Input: part model. Units: mm. Frame: model coordinates. Face numbers are marked on the shaded views. Round coordinates to 2 decimals unless told otherwise and drop trailing zeros. Write each loop counter-clockwise with the first axis right and the second up, starting at its lowest first coordinate (ties: lowest second). Pieces come first, ordered by that corner, then holes. Notation, with made-up numbers: (57.25, 86.25) -> (72.25, 86.25) arc R21 ccw to (72.25, 119.25) -> close; hole circle Ø9 at (-5.5, 19). An arc over 180 degrees is marked (long way). Write item = value, one per line.
```python
from build123d import *

# Parameters (mm, degrees)
SKETCH1_R           = 25
BOSS_EXTRUDE1_DEPTH = 29.5
SKETCH2_R           = 40
BOSS_EXTRUDE2_DEPTH = 3
CHAMFER1_SIZE       = 1
SKETCH3_R           = 21
CUT_EXTRUDE1_DEPTH  = 26
FILLET1_R           = 0.5
SKETCH4_R           = 2
CUT_EXTRUDE2_DEPTH  = 26
CIRPATTERN1_COUNT   = 4
CHAMFER2_SIZE       = 0.5


with BuildPart() as part:
    # Sketch1 → Boss-Extrude1 (new body)
    with BuildSketch(Plane.XY):
        Circle(SKETCH1_R)
    extrude(amount=BOSS_EXTRUDE1_DEPTH)

    # Sketch2 → Boss-Extrude2 (add)
    with BuildSketch(Plane.XY.offset(29.5)):
        Circle(SKETCH2_R)
    extrude(amount=-BOSS_EXTRUDE2_DEPTH)

    # Chamfer1
    chamfer1_edges = [part.edges().sort_by_distance(p)[0] for p in [
        (-25, 0, 0),
        (-25, 0, 26.5),
    ]]
    chamfer(chamfer1_edges, length=CHAMFER1_SIZE)

    # Sketch3 → Cut-Extrude1 (cut)
    with BuildSketch(Plane.XY.offset(29.5)):
        Circle(SKETCH3_R)
    extrude(amount=-CUT_EXTRUDE1_DEPTH, mode=Mode.SUBTRACT)

    # Fillet1
    fillet1_edges = [part.edges().sort_by_distance(p)[0] for p in [
        (-40, 0, 26.5),
        (-40, 0, 29.5),
    ]]
    fillet(fillet1_edges, radius=FILLET1_R)

    # Sketch4 → Cut-Extrude2 (cut)
    with BuildSketch(Plane(origin=(0, 0, 26.5), x_dir=(-1, 0, 0), z_dir=(0, 0, -1))):
        with Locations((0, 32.5)):
            Circle(SKETCH4_R)
    cut_extrude2 = extrude(amount=-CUT_EXTRUDE2_DEPTH, mode=Mode.SUBTRACT)

    # CirPattern1: Cut-Extrude2 ×4 about axis
    cirpattern1_axis = Axis((0, 0, 0), (0, 0, 1))
    for i in range(1, CIRPATTERN1_COUNT):
        add(cut_extrude2.rotate(cirpattern1_axis, i * 360 / CIRPATTERN1_COUNT), mode=Mode.SUBTRACT)

    # Chamfer2
    chamfer2_edges = [part.edges().sort_by_distance(p)[0] for p in [
        (2, 32.5, 26.5),
        (32.5, -2, 26.5),
        (-2, -32.5, 29.5),
        (-2, -32.5, 26.5),
        (-32.5, 2, 26.5),
    ]]
    chamfer(chamfer2_edges, length=CHAMFER2_SIZE)


solid = part.part
```
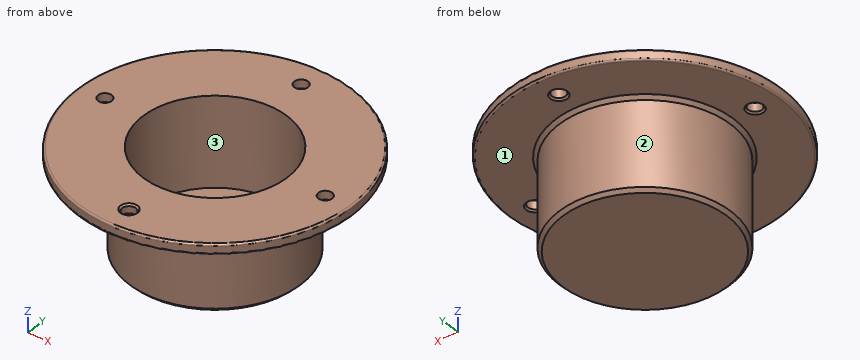
1) Line query: L1, parallel to Y at x = 0, z = 28; L2, parallel to Y at x = -0.5, z = 27.25; L3, parallel to Z at x = -15, y = -4. Output: solid intervals per line, ascending. Write a range as from..to.
Solutions:
L1 = -40..-34.5, -30.5..-21, 21..30.5, 34.5..40
L2 = -40..-34.44, -30.56..-20.99, 20.99..30.56, 34.44..40
L3 = 0..3.5
2) Draft query along Y for the marked faces 1, 2 and 3. Return one class per face: +Y half, -Y half, draft (parallel to the pull), parting line (faces both ways), or undercut.
Solutions:
face_1 = draft
face_2 = parting line
face_3 = undercut
3) First-contact query: P1, Ø5, axis at x = 2, z = 9, coming from the -Y side; P2, Ø6.5, axis at x = 0, y = -32.5, coming from the -Z side; P3, Ø3, axis at x = 32.5, y = 0, coming from the -Z side; P4, Ø8, axis at y = 26.5, z = 4, coming from the +X side. Flat tips, straight axial feed; report the tip coordinate or a pass-through.
Solutions:
P1 = -25
P2 = 26.5
P3 = through
P4 = 10.9
4) Cut plane A-A (x = 0). Count the separate pieces of the cut face and the enclosed holes in it, and give its area (3 significant figures).
Solutions:
separate_pieces = 3
enclosed_holes = 0
area = 448 mm^2
5) Cut plane C-C (z = 18.5). Return the cut outline in (x, y), and give its area (3 significant figures).
Solutions:
outline = circle Ø50 at (0, 0); hole circle Ø42 at (0, 0)
area = 578 mm^2
